Model file for the job. Use its own axes, mm. A direction names the side the tool comes from. Give positions to 0.01 mm unless a question says otherwise; leave off trailing zeros. Loops run counter-clockwise (first coordinate to the right, second up) from the corner with the lowest first, then second, coordinate; pieces in that order, holes last. Notation, with made-up numbers: M 81,13.5 L 131,13.5 A11 ccw 131,21.5 Z; hole C 13,67 d10. An arc over 180 degrees is marked long. Answer in a Markdown table with one row per item.
```python
from build123d import *

# Parameters (mm, degrees)
SKETCH_1_W      = 4
SKETCH_1_H      = 13
SKETCH_1_W_2    = 9
SKETCH_1_W_3    = 5.5
SKETCH_1_W_4    = 7
EXTRUDE_1_DEPTH = 3
FILLET_1_R      = 0.5
FILLET_2_R      = 1


with BuildPart() as part:
    # Эскиз1 → Бобышка-Вытянуть1 (new body)
    with BuildSketch(Plane(origin=(0, 0, 0), x_dir=(1, 0, 0), z_dir=(0, 1, 0))):
        Polygon((-56.25, -11.4), (56.25, -11.4), (56.25, -5.65), (59.25, -5.65), (59.25, 4.35), (56.25, 4.35), (56.25, 9.6), (-56.25, 9.6), (-56.25, 4.35), (-59.25, 4.35), (-59.25, -5.65), (-56.25, -5.65), align=None)
        with Locations((-41.75, 0)):
            Rectangle(SKETCH_1_W, SKETCH_1_H, mode=Mode.SUBTRACT)
        with Locations((39.25, 0)):
            Rectangle(SKETCH_1_W_2, SKETCH_1_H, mode=Mode.SUBTRACT)
        with Locations((-23.625, 0)):
            Rectangle(SKETCH_1_W_3, SKETCH_1_H, mode=Mode.SUBTRACT)
        with Locations((-33.0625, 0)):
            Rectangle(SKETCH_1_W_3, SKETCH_1_H, mode=Mode.SUBTRACT)
        with Locations((-14.1875, 0)):
            Rectangle(SKETCH_1_W_3, SKETCH_1_H, mode=Mode.SUBTRACT)
        with Locations((-4.75, 0)):
            Rectangle(SKETCH_1_W_3, SKETCH_1_H, mode=Mode.SUBTRACT)
        with Locations((16.375, 0)):
            Rectangle(SKETCH_1_W_4, SKETCH_1_H, mode=Mode.SUBTRACT)
        with Locations((5.4375, 0)):
            Rectangle(SKETCH_1_W_4, SKETCH_1_H, mode=Mode.SUBTRACT)
        with Locations((27.3125, 0)):
            Rectangle(SKETCH_1_W_4, SKETCH_1_H, mode=Mode.SUBTRACT)
    extrude(amount=EXTRUDE_1_DEPTH)

    # Скругление1
    fillet_1_edges = [part.edges().sort_by_distance(p)[0] for p in [
        (-59.25, 1.5, 5.65),
        (-59.25, 1.5, -4.35),
        (59.25, 1.5, -4.35),
        (59.25, 1.5, 5.65),
    ]]
    fillet(fillet_1_edges, radius=FILLET_1_R)

    # Скругление2
    fillet_2_edges = [part.edges().sort_by_distance(p)[0] for p in [
        (-56.25, 1.5, -9.6),
        (56.25, 1.5, -9.6),
        (56.25, 1.5, 11.4),
        (-56.25, 1.5, 11.4),
    ]]
    fillet(fillet_2_edges, radius=FILLET_2_R)


solid = part.part
```
Q1. Probe probe 1 along Z at (x, y) = (-6, 0.25); probe 2 along X at (y, z) = (0.7, 8.25). List the from-to ranges inside material, lowest first.
Reported:
| item | result |
|---|---|
| probe 1 | -9.6 to -6.5, 6.5 to 11.4 |
| probe 2 | -56.25 to 56.25 |
Q2. Saw through at B-B (z = 0.5). Give the number of separate pieces and of enclosed holes in the cut face, and give its area (4 significant figures).
Reported:
| item | result |
|---|---|
| separate pieces | 10 |
| enclosed holes | 0 |
| area | 187.5 mm² |
Q3. 3-axis set-ups, long thin cutter, end or side, ignore diameter. For faces 4 (the face through (-1, 0, 1)), 5 (the face through (5, 1, 6.5)), 6 (the face through (-58, 1, 5.65)): which of +Z, -Z, +X, -X, +Y, -Y reach the whole face in a straight line?
Reported:
| item | result |
|---|---|
| face 4 | +Z, -Z, +X, -X, -Y |
| face 5 | +Y, -Y |
| face 6 | +Z, -X, +Y, -Y |
Q4. Saw through at A-A (x = -41). Give the cut face in (y, z), and give its area (3 significant figures).
Reported:
| item | result |
|---|---|
| outline | M 0,-9.6 L 3,-9.6 L 3,-6.5 L 0,-6.5 Z; M 0,6.5 L 3,6.5 L 3,11.4 L 0,11.4 Z |
| area | 24.0 mm² |
Q5. Saw through at D-D (z = 8.5). Give the cut face in (x, y), and give its area (4 significant figures).
Reported:
| item | result |
|---|---|
| outline | M -56.25,0 L 56.25,0 L 56.25,3 L -56.25,3 Z |
| area | 337.5 mm² |
Q6. Drop flat-ended pins along their axis: pin 1 (1 mm diameter, centred on x = -12, z = 5.5, fed in from -Y); pin 2 (0.9 mm diameter, centred on y = 1.5, z = -5.5, fed in from +X). Give the stop position or say it passes through.
Reported:
| item | result |
|---|---|
| pin 1 | through |
| pin 2 | x = 56.25 |
Q7. Mould opens along X. For faces 1 (the face through (-59.25, 1, 1)), 2 (the face through (1.938, 1, 0)), 3 (the face through (56.25, 1, -6)) say: released by +X, released by -X, zero draft, split by the parting line, or undercut.
Reported:
| item | result |
|---|---|
| face 1 | released by -X |
| face 2 | undercut |
| face 3 | released by +X |
